Geometry: final body of the model. Coordinates: model frame, mm. Face numbers are marked on the shaded views. Give positions to 0.01 mm unless a question says otherwise; leave off trailing zeros. Loops run counter-clockwise (first coordinate to the right, second up) from the corner with the lowest first, then second, coordinate; pieces in that order, holes last. Notation, with made-up numbers: (-15.75, -15) -> (37.25, -15) arc R20 cw to (37.25, -9) -> close; hole circle Ø5 at (22, 68). An arc over 180 degrees is marked (long way). One line per question, with ' | ' between items. Start each with the question number.
Item 1: Section B-B on x = 4. Return loops of the section in (y, z), then the cut area to 3 significant figures.
Item 2: Pin query (flat end, axial travel): P1, Ø1.8, axis at x = 4, z = 2.5, coming from the -Y side; P2, Ø1.5, axis at y = 17, z = 3, coming from the -X side; P3, Ø1, axis at y = 14, z = 4, coming from the -X side. Return the tip coordinate at first contact, or that it passes through.
Item 3: Mould query, pull axis Y, two halves, no side actions, for the marked faces 1, 2 and 3. Classes: released by +Y, released by -Y, zero draft, split by the parting line, or undercut.
Item 4: Section C-C on y = 15. Return loops of the section in (x, z), then the cut area to 3 significant figures.
Item 5: Material intervals for line 1 along Y through (x, z) = (40, 2); line 2 along X through (y, z) = (15.25, 4.45); line 3 along Z through (x, y) = (4, 28.6), sorted ascending. Write a range as [from, to].
Item 6: Section D-D on y = 2. Return loops of the section in (x, z).
Item 7: Section A-A on z = 2.5. Give the number of separate pieces and of enclosed holes in the cut face, then the cut area to 3 significant figures.
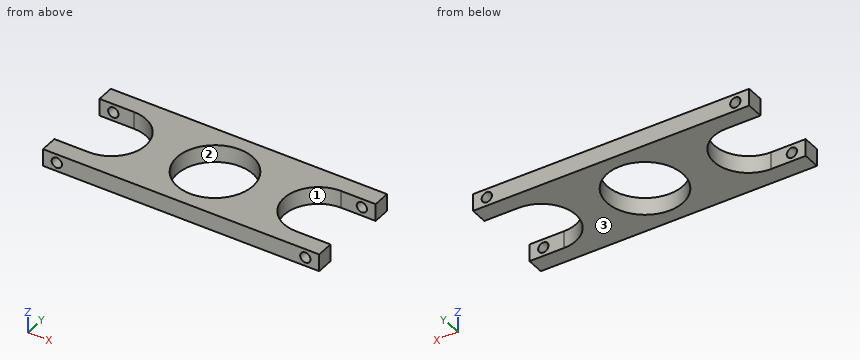
from build123d import *

# Parameters (mm, degrees)
ESQUISSE1_R        = 11
BOSS_EXTRU_1_DEPTH = 5
D_GAGEMENT_M31_D   = 3


with BuildPart() as part:
    # Esquisse1 → Boss.-Extru.1 (new body)
    with BuildSketch(Plane.XY):
        with BuildLine():
            Line((0, 0), (80, 0))
            Line((80, 0), (80, 5))
            Line((80, 5), (70, 5))
            ThreePointArc((70, 5), (60, 15), (70, 25))
            Line((70, 25), (80, 25))
            Line((80, 25), (80, 30))
            Line((80, 30), (0, 30))
            Line((0, 30), (0, 25))
            Line((0, 25), (10, 25))
            ThreePointArc((10, 25), (20, 15), (10, 5))
            Line((10, 5), (0, 5))
            Line((0, 5), (0, 0))
        make_face()
        with Locations((40, 15)):
            Circle(ESQUISSE1_R, mode=Mode.SUBTRACT)
    extrude(amount=BOSS_EXTRU_1_DEPTH)

    # Dégagement M31 (through all)
    with Locations(Plane(origin=(0, 30, 0), x_dir=(1, 0, 0), z_dir=(0, 1, 0))):
        with Locations((4, -2.5), (76, -2.5)):
            Hole(D_GAGEMENT_M31_D / 2)


solid = part.part
Result sheet:
1) outline: (0, 0) -> (5, 0) -> (5, 1) -> (0, 1) -> close; (0, 4) -> (5, 4) -> (5, 5) -> (0, 5) -> close; (25, 0) -> (30, 0) -> (30, 1) -> (25, 1) -> close; (25, 4) -> (30, 4) -> (30, 5) -> (25, 5) -> close | area: 20.0 mm²
2) P1: passes through | P2: stops at x = 19.61 | P3: stops at x = 19.89
3) face 1: undercut | face 2: undercut | face 3: zero draft
4) outline: (20, 0) -> (29, 0) -> (29, 5) -> (20, 5) -> close; (51, 0) -> (60, 0) -> (60, 5) -> (51, 5) -> close | area: 90.0 mm²
5) line 1: y = [0, 4], [26, 30] | line 2: x = [20, 29], [51, 60] | line 3: z = [0, 1], [4, 5]
6) outline: (0, 0) -> (80, 0) -> (80, 5) -> (0, 5) -> close; hole circle Ø3 at (4, 2.5); hole circle Ø3 at (76, 2.5)
7) separate pieces: 5 | enclosed holes: 1 | area: 1,250 mm²
